Could you check a few things on this model? Use its own coordinates, in mm. Face numbers are marked on the shaded views. A direction names the side the tool comes from. Round coordinates to 2 decimals unless told otherwise and drop trailing zeros. Order: outer loops, then holes, each group sorted by start corner. A loop starts at its lowest first (then second) coordinate and runs counter-clockwise, first axis right, second up. Notation, with made-up numbers: (-33.5, 60.5) -> (15.5, 60.5) arc R24 ccw to (15.5, 77.5) -> close; hole circle Ø4 at (72.5, -18). An arc over 180 degrees is marked (long way). One line per question, with ' | ' between items.
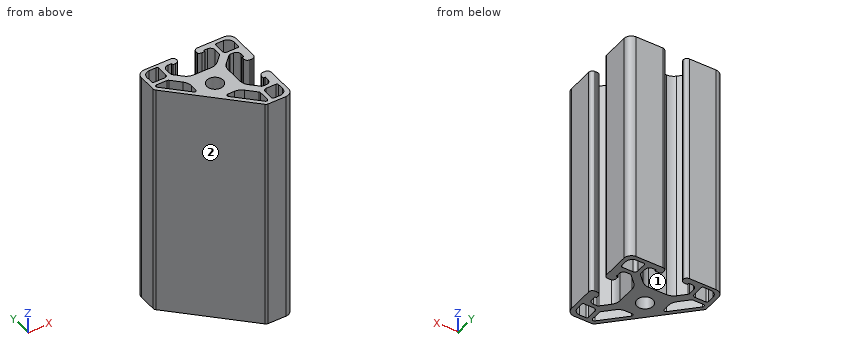
Autodesk Inventor part; units mm, degrees
ref_plane "YZ Plane" through (0, 0, 0) normal (1, 0, 0) x (0, 1, 0)
ref_plane "XZ Plane" through (0, 0, 0) normal (0, 1, 0) x (-1, 0, 0)
ref_plane "XY Plane" through (0, 0, 0) normal (0, 0, 1) x (1, 0, 0)
sketch "Sketch1" plane through (0, 0, 0) normal (0, 0, 1) x (1, 0, 0)
  circle A0 centre (0, 0) radius 3.4
  arc A1 (-13.205, 12.2693) -> (-11.935, 13.5393) centre (-13.205, 13.5393) ccw
  line L0 (-17.695, 12.2693) -> (-13.205, 12.2693)
  arc A2 (-18.325, 12.8993) -> (-17.695, 12.2693) centre (-17.695, 12.8993) ccw
  line L1 (-18.325, 15.8793) -> (-18.325, 12.8993)
  arc A3 (-15.525, 18.6793) -> (-18.325, 15.8793) centre (-15.525, 15.8793) ccw
  line L2 (-12.565, 18.6793) -> (-15.525, 18.6793)
  arc A4 (-11.935, 18.0493) -> (-12.565, 18.6793) centre (-12.565, 18.0493) ccw
  line L3 (-11.935, 13.5393) -> (-11.935, 18.0493)
  arc A5 (-7.7004, 3.4003) -> (-9.0909, 6.7575) centre (-12.4481, 3.4003) ccw
  line L4 (-7.7004, 0.5997) -> (-7.7004, 3.4003)
  arc A6 (-8.9978, 0.0623) -> (-7.7004, 0.5997) centre (-8.4604, 0.5997) ccw
  line L5 (-18.2574, 9.3219) -> (-8.9978, 0.0623)
  arc A7 (-17.72, 10.6193) -> (-18.2574, 9.3219) centre (-17.72, 9.8593) ccw
  line L6 (-13.3072, 10.6193) -> (-17.72, 10.6193)
  arc A8 (-12.7021, 10.3687) -> (-13.3072, 10.6193) centre (-13.3072, 9.7636) ccw
  line L7 (-9.0909, 6.7575) -> (-12.7021, 10.3687)
  arc A9 (10.5703, -13.2185) -> (10.3477, -12.6811) centre (9.8103, -13.2185) ccw
  line L8 (10.5703, -17.6313) -> (10.5703, -13.2185)
  arc A10 (9.2729, -18.1687) -> (10.5703, -17.6313) centre (9.8103, -17.6313) ccw
  line L9 (-0.0445, -8.8513) -> (9.2729, -18.1687)
  arc A11 (0.4929, -7.5539) -> (-0.0445, -8.8513) centre (0.4929, -8.3139) ccw
  line L10 (3.2583, -7.5539) -> (0.4929, -7.5539)
  arc A12 (6.6079, -8.9413) -> (3.2583, -7.5539) centre (3.2583, -12.2908) ccw
  line L11 (10.3477, -12.6811) -> (6.6079, -8.9413)
  arc A13 (12.2693, -17.72) -> (12.8993, -18.35) centre (12.8993, -17.72) ccw
  line L12 (12.2693, -13.5393) -> (12.2693, -17.72)
  arc A14 (13.5393, -12.2693) -> (12.2693, -13.5393) centre (13.5393, -13.5393) ccw
  line L13 (17.72, -12.2693) -> (13.5393, -12.2693)
  arc A15 (18.35, -12.8993) -> (17.72, -12.2693) centre (17.72, -12.8993) ccw
  line L14 (18.35, -15.55) -> (18.35, -12.8993)
  arc A16 (15.55, -18.35) -> (18.35, -15.55) centre (15.55, -15.55) ccw
  line L15 (12.8993, -18.35) -> (15.55, -18.35)
  arc A17 (12.565, 18.332) -> (11.935, 17.702) centre (12.565, 17.702) ccw
  line L16 (15.55, 18.332) -> (12.565, 18.332)
  arc A18 (18.35, 15.532) -> (15.55, 18.332) centre (15.55, 15.532) ccw
  line L17 (18.35, 12.8413) -> (18.35, 15.532)
  arc A19 (17.745, 12.2693) -> (18.35, 12.8413) centre (17.7226, 12.8989) ccw
  line L18 (13.205, 12.2693) -> (17.745, 12.2693)
  arc A20 (11.935, 13.5393) -> (13.205, 12.2693) centre (13.205, 13.5393) ccw
  line L19 (11.935, 17.702) -> (11.935, 13.5393)
  arc A21 (8.04, -3.74) -> (9.4306, -7.0971) centre (12.7878, -3.74) ccw
  line L20 (8.04, -3.74) -> (8.04, 3.74)
  arc A22 (9.4306, 7.0971) -> (8.04, 3.74) centre (12.7878, 3.74) ccw
  line L21 (9.4306, 7.0971) -> (12.6921, 10.3586)
  arc A23 (13.3214, 10.6193) -> (12.6921, 10.3586) centre (13.3214, 9.7293) ccw
  line L22 (13.3214, 10.6193) -> (14.8088, 10.6193)
  arc A24 (16.7, 8.7281) -> (14.8088, 10.6193) centre (14.8088, 8.7281) ccw
  line L23 (16.7, 8.7281) -> (16.7, 6.9134)
  line L24 (16.7, 6.9134) -> (15.94, 6.9134)
  line L25 (15.94, 6.9134) -> (15.94, 5.7595)
  arc A25 (15.94, 5.7595) -> (17.51, 4.1895) centre (17.51, 5.7595) ccw
  line L26 (17.51, 4.1895) -> (18.43, 4.1895)
  arc A26 (18.43, 4.1895) -> (20, 5.7595) centre (18.43, 5.7595) ccw
  line L27 (20, 5.7595) -> (20, 16.8689)
  arc A27 (20, 16.8689) -> (16.8881, 20) centre (16.8302, 16.8305) ccw
  line L28 (16.8881, 20) -> (5.6295, 20)
  arc A28 (5.6295, 20) -> (4.06, 18.4701) centre (5.6295, 18.43) ccw
  line L29 (4.06, 18.4701) -> (4.06, 17.5501)
  arc A29 (4.06, 17.5501) -> (5.63, 16.8567) centre (5.3762, 18.406) ccw
  line L30 (5.63, 16.8567) -> (6.7535, 16.8567)
  line L31 (6.7535, 16.8567) -> (6.7535, 17.6167)
  line L32 (6.7535, 17.6167) -> (8.3698, 17.6167)
  arc A30 (10.285, 15.7015) -> (8.3698, 17.6167) centre (8.3698, 15.7015) ccw
  line L33 (10.285, 15.7015) -> (10.285, 12.8154)
  arc A31 (10.2371, 12.5705) -> (10.285, 12.8154) centre (9.6352, 12.8154) ccw
  line L34 (10.2371, 12.5705) -> (7.0971, 9.4306)
  arc A32 (3.74, 8.04) -> (7.0971, 9.4306) centre (3.74, 12.7878) ccw
  line L35 (3.74, 8.04) -> (-3.74, 8.04)
  arc A33 (-7.0971, 9.4306) -> (-3.74, 8.04) centre (-3.74, 12.7878) ccw
  line L36 (-7.0971, 9.4306) -> (-10.0289, 12.3623)
  arc A34 (-10.285, 12.9807) -> (-10.0289, 12.3623) centre (-9.4106, 12.9807) ccw
  line L37 (-10.285, 12.9807) -> (-10.285, 15.7015)
  arc A35 (-8.3698, 17.6167) -> (-10.285, 15.7015) centre (-8.3698, 15.7015) ccw
  line L38 (-8.3698, 17.6167) -> (-6.7535, 17.6167)
  line L39 (-6.7535, 17.6167) -> (-6.7535, 16.8567)
  line L40 (-6.7535, 16.8567) -> (-5.63, 16.8567)
  arc A36 (-5.63, 16.8567) -> (-4.06, 18.4267) centre (-5.63, 18.4267) ccw
  line L41 (-4.06, 18.4267) -> (-4.06, 18.4153)
  arc A37 (-4.06, 18.4153) -> (-5.6299, 20) centre (-5.6299, 18.43) ccw
  line L42 (-5.6299, 20) -> (-16.83, 20)
  arc A38 (-16.83, 20) -> (-20, 16.83) centre (-16.83, 16.83) ccw
  line L43 (-20, 16.83) -> (-20, 9.3524)
  arc A39 (-20, 9.3524) -> (-19.5607, 8.2917) centre (-18.5, 9.3524) ccw
  line L44 (-19.5607, 8.2917) -> (8.2917, -19.5607)
  arc A40 (8.2917, -19.5607) -> (9.3524, -20) centre (9.3524, -18.5) ccw
  line L45 (9.3524, -20) -> (16.83, -20)
  arc A41 (16.83, -20) -> (20, -16.83) centre (16.83, -16.83) ccw
  line L46 (20, -16.83) -> (20, -5.7595)
  arc A42 (20, -5.7595) -> (18.43, -4.1895) centre (18.43, -5.7595) ccw
  line L47 (18.43, -4.1895) -> (17.51, -4.1895)
  arc A43 (17.51, -4.1895) -> (15.94, -5.7595) centre (17.51, -5.7595) ccw
  line L48 (15.94, -5.7595) -> (15.94, -6.9134)
  line L49 (15.94, -6.9134) -> (16.7, -6.9134)
  line L50 (16.7, -6.9134) -> (16.7, -8.7281)
  arc A44 (14.8088, -10.6193) -> (16.7, -8.7281) centre (14.8088, -8.7281) ccw
  line L51 (14.8088, -10.6193) -> (13.3214, -10.6193)
  arc A45 (12.6921, -10.3586) -> (13.3214, -10.6193) centre (13.3214, -9.7293) ccw
  line L52 (12.6921, -10.3586) -> (9.4306, -7.0971)
extrude "Extrusion1" add sketch "Sketch1" against normal blind 100
properties part number "40-4045-LITE-BLACK-FB"
1. I need wall thicknesses on probe 1 along Y at (x, z) = (0, -32.5); probe 2 along X at (y, z) = (-9.5, -18.5); probe 3 along Y at (x, z) = (13, -10). Which ranges of each line are inside material? Lowest first, please.
From the geometry:
probe 1: y = -11.27 to -8.9, -7.74 to -3.4, 3.4 to 8.04 | probe 2: x = -1.77 to 0.6, 7.17 to 11.83, 16.54 to 20 | probe 3: y = -20 to -18.35, -12.39 to -10.56, 10.56 to 12.29, 18.33 to 20
2. On a 3-axis mill with a long thin cutter (end or side, diameter ignored), from which of +Z, -Z, +X, -X, +Y, -Y can I reach the whole of each face in a straight line? I mean the marked faces 1 and 2. Say none if no direction works.
From the geometry:
face 1: +Z, -Z, +Y | face 2: +Z, -Z, -X, -Y
3. I want a section at A-A on x = 2. List the corners of the cut face in (y, z) for me.
From the geometry:
outline: (-13.27, -100) -> (-10.9, -100) -> (-10.9, 0) -> (-13.27, 0) -> close; (-7.55, -100) -> (-2.75, -100) -> (-2.75, 0) -> (-7.55, 0) -> close; (2.75, -100) -> (8.04, -100) -> (8.04, 0) -> (2.75, 0) -> close
4. I want a section at B-B on z = -59.5. Count the separate pieces of the cut face and the enclosed holes in it, and give its area (3 significant figures).
From the geometry:
separate pieces: 1 | enclosed holes: 6 | area: 551 mm²
5. I'm going to push flat-ended pins straight in: pin 1 (8 mm diameter, centred on x = -12.5, z = -41.5, fed in from -Y); pin 2 (6 mm diameter, centred on y = -0.5, z = -34, fed in from +X); pin 3 (1 mm diameter, centred on x = 6, y = -12.5, fed in from -Z); pin 4 (1.8 mm diameter, centred on x = 7.5, z = -32.5, fed in from -Y). Where does each tip first touch, or does it pass through?
From the geometry:
pin 1: stops at y = -2.77 | pin 2: stops at x = 8.04 | pin 3: passes through | pin 4: stops at y = -19.66
